Check sheet for the drawn part. Datum: minimum x, y, z corner. Units: mm. Give positions to 0.01 mm unless a question says otherwise; leave off trailing zeros. Write each loop counter-clockwise with the first axis right and the second up, starting at its lowest first coordinate (ties: lowest second). Pieces come first, ordered by that corner, then holes. Notation, with made-up numbers: (-7, -17) - (37, -17) arc R31 cw to (37, 12) - close; hole circle Ø3 at (80.5, -9.5). An arc over 180 degrees is marked (long way). Answer as a JSON object with one key per item and string values. Group by question number.
Item 1: Go/stop test with flat-tipped pins: pin 1 (2.5 mm diameter, centred on y = 2, z = 131, fed in from +X); pin 2 (2.5 mm diameter, centred on x = 13.5, y = 3, fed in from +Z); pin 3 (2.5 mm diameter, centred on y = 2.5, z = 18, fed in from -X). Record where each tip stops, or that it passes through.
Item 2: Scan line: line 1 along X through (y, z) = (3.4, 136). Record every from-to range of solid material in increasing order. Write a range as [from, to].
Item 3: Sectioned sample at A-A, the plane y = 2.75. Record the boundary of the cut face in (x, z), and give its area (3 significant figures).
Item 4: Sectioned sample at B-B, the plane z = 117.5. Record the boundary of the cut face in (x, y), and give its area (4 significant figures).
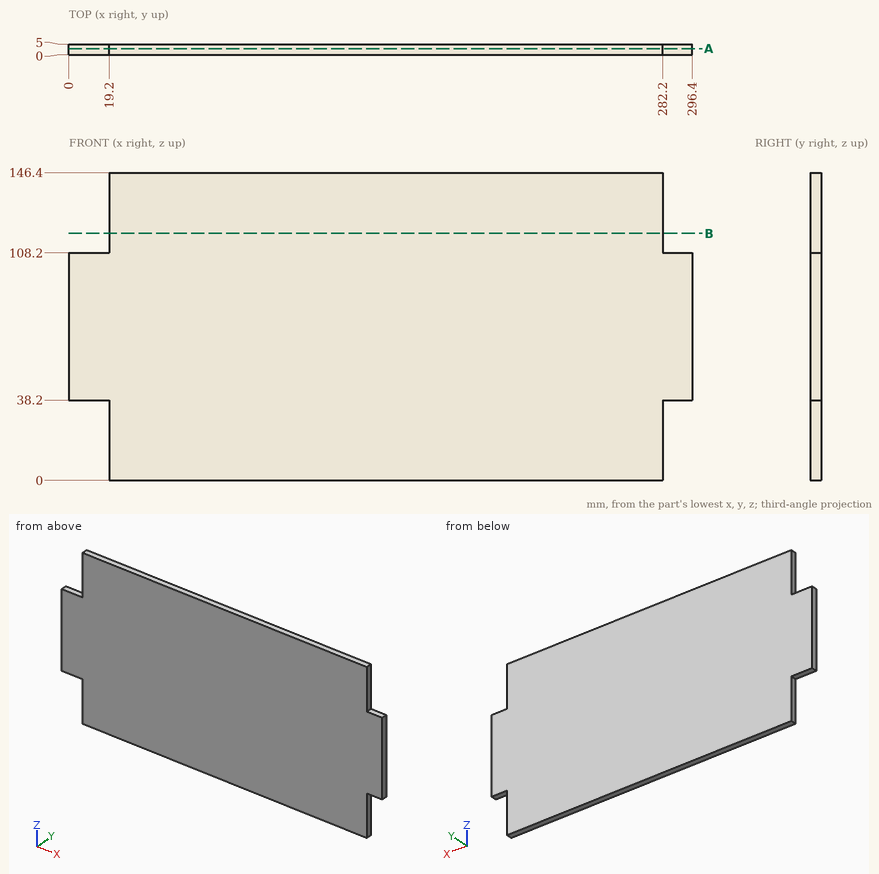
Geometry check:
{
 "1": {"pin 1": "x = 282.2", "pin 2": "z = 108.2", "pin 3": "x = 19.2"},
 "2": {"line 1": "[19.2, 282.2]"},
 "3": {"outline": "(0, 38.2) - (19.2, 38.2) - (19.2, 0) - (282.2, 0) - (282.2, 38.2) - (296.4, 38.2) - (296.4, 108.2) - (282.2, 108.2) - (282.2, 146.4) - (19.2, 146.4) - (19.2, 108.2) - (0, 108.2) - close", "area": "40,800 mm^2"},
 "4": {"outline": "(19.2, 0) - (282.2, 0) - (282.2, 5) - (19.2, 5) - close", "area": "1,315 mm^2"}
}
